The listing builds one solid part. Answer for the finished solid, in the listing's coordinates (mm). Coordinates: 2 decimals unless noted, no trailing zeros. Write each loop counter-clockwise with the first axis right and the second up, starting at its lowest first coordinate (ties: lowest second). Pieces come first, ordered by that corner, then holes. Notation, with made-up numbers: M 4.25,31 L 33.25,31 A6 ccw 33.25,39 Z; hole C 49,76.25 d7. An arc over 180 degrees is marked long. Answer as CSV lines item,"result". Start each with the question number.
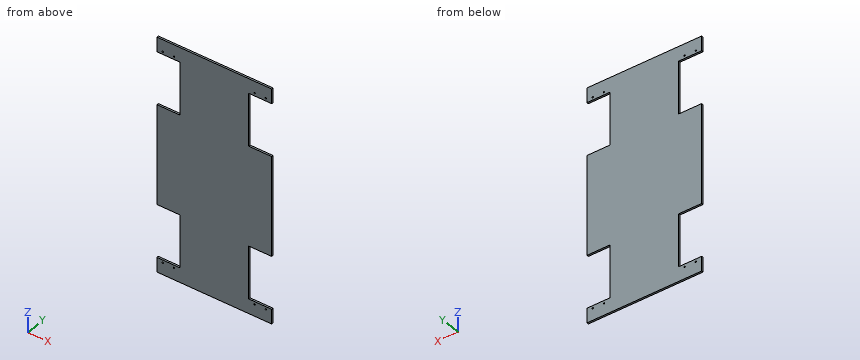
```python
from build123d import *

# Parameters (mm, degrees)
BOSS_EXTRUDE1_DEPTH                  = 3.175
F_3_32_0_09375_DIAMETER_HOLE1_D      = 2.38125
MIRROR5_AT_THE_SECOND_PLANE_COPY_1_D = 2.38125


with BuildPart() as part:
    # Sketch1 → Boss-Extrude1 (new body)
    with BuildSketch(Plane(origin=(0, 0, 0), x_dir=(1, 0, 0), z_dir=(0, 1, 0))):
        Polygon((-100, 85), (-100, -85), (-60, -85), (-60, -175), (-100, -175), (-100, -200), (100, -200), (100, -175), (60, -175), (60, -85), (100, -85), (100, 85), (60, 85), (60, 175), (100, 175), (100, 200), (-100, 200), (-100, 175), (-60, 175), (-60, 85), align=None)
    extrude(amount=BOSS_EXTRUDE1_DEPTH)

    # 3/32 (0.09375) Diameter Hole1 (through all)
    with Locations(Plane(origin=(0, 3.175, 0), x_dir=(1, 0, 0), z_dir=(0, 1, 0))):
        with Locations((-89.78, 179.7625), (-70.22, 179.7625)):
            f_3_32_0_09375_diameter_hole1 = Hole(F_3_32_0_09375_DIAMETER_HOLE1_D / 2)

    # Mirror5: 3/32 (0.09375) Diameter Hole1 across plane
    add(f_3_32_0_09375_diameter_hole1.mirror(Plane(origin=(0, 0, 0), x_dir=(0, 0, 1), z_dir=(1, 0, 0))), mode=Mode.SUBTRACT)

    # Mirror5 at the second plane: 3/32 (0.09375) Diameter Hole1 across plane
    add(f_3_32_0_09375_diameter_hole1.mirror(Plane.XY), mode=Mode.SUBTRACT)

    # Mirror5 at the second plane copy 1 (through all)
    with Locations(Plane(origin=(0, 3.175, 0), x_dir=(-1, 0, 0), z_dir=(0, 1, 0))):
        with Locations((-89.78, 179.7625), (-70.22, 179.7625)):
            Hole(MIRROR5_AT_THE_SECOND_PLANE_COPY_1_D / 2)


solid = part.part
```
1) The part is cut by section A-A (y = 2.35). Count the separate pieces of the cut face and the enclosed holes in it, then the cut area to 3 significant figures.
2) Each of these flat-tipped pins is pushed along its axis until it touches: P1, Ø1, axis at y = 1, z = -135.5, coming from the -X side; P2, Ø1, axis at y = 1, z = 129.5, coming from the +X side; P3, Ø1.9, axis at x = 70.22, z = 179.76, coming from the -Y side (3 decimals). Where does it stop, or does it pass through?
3) Find the intervals of material crossed by line 1 (Z direction, x = 68.5, y = 0.5); line 2 (Z direction, x = 89.78, y = 1.25); line 3 (X direction, y = 2.1, z = 150), in increasing order. Write a range as from..to.
4) The part is cut by section B-B (z = 110.5). Determine the outline of the cut face in (x, y) (3 decimals), then the cut area to 3 significant figures.
Completed:
1,separate pieces,"1"
1,enclosed holes,"8"
1,area,"65,600 mm²"
2,P1,"x = -60"
2,P2,"x = 60"
2,P3,"through"
3,line 1,"-200..-175, -85..85, 175..200"
3,line 2,"-200..-180.95, -178.57..-175, -85..85, 175..178.57, 180.95..200"
3,line 3,"-60..60"
4,outline,"M -60,0 L 60,0 L 60,3.175 L -60,3.175 Z"
4,area,"381 mm²"
